```python
from build123d import *

# Parameters (mm, degrees)
F2_R     = 25.25
F3_DEPTH = 18
F4_R     = 23
F5_DEPTH = 2
F6_R     = 30.25
F6_R_2   = 25.25
F7_DEPTH = 12
F9_D     = 2
F9_DEPTH = 5
F9_TIP   = 0.600860619


with BuildPart() as f1:
    # F0 (on Right) → F1 (revolve)
    with BuildSketch(Plane.YZ):
        Polygon((0, 41), (0, 0), (20, 0), (20, 41), (16, 41), (16, 35), (12, 35), (6, 41), align=None)
    revolve(axis=Axis((0, 10, 0), (0, -1, 0)))

    # F2 (on face) → F3 (cut)
    with BuildSketch(Plane(origin=(0, 20, 0), x_dir=(-1, 0, 0), z_dir=(0, 1, 0))):
        Circle(F2_R)
    extrude(amount=-F3_DEPTH, mode=Mode.SUBTRACT)

    # F4 (on face) → F5 (cut, through all)
    with BuildSketch(Plane.XZ):
        Circle(F4_R)
    extrude(amount=-F5_DEPTH, mode=Mode.SUBTRACT)

    # F6 (on face) → F7 (cut)
    with BuildSketch(Plane(origin=(0, 20, 0), x_dir=(-1, 0, 0), z_dir=(0, 1, 0))):
        Circle(F6_R)
        Circle(F6_R_2, mode=Mode.SUBTRACT)
    extrude(amount=-F7_DEPTH, mode=Mode.SUBTRACT)

    # F9
    with Locations(Plane(origin=(0, 8, 0), x_dir=(-1, 0, 0), z_dir=(0, 1, 0))):
        with Locations((0, 27.75), (24.032204955, -13.875), (-24.032204955, -13.875)):
            Hole(F9_D / 2, depth=F9_DEPTH)
            with Locations((0, 0, -(F9_DEPTH + F9_TIP / 2))):  # 118° drill point
                Cone(0, F9_D / 2, F9_TIP, mode=Mode.SUBTRACT)


solid = f1.part
```
The listing builds one solid part. Answer for the finished solid, in the listing's coordinates (mm). A direction names the side the tool comes from. Give positions to 0.01 mm unless a question says otherwise; leave off trailing zeros. Order: outer loops, then holes, each group sorted by start corner. A loop starts at its lowest first (then second) coordinate and runs counter-clockwise, first axis right, second up. Notation, with made-up numbers: (22.25, 56.5) -> (72.25, 56.5) arc R14 ccw to (72.25, 62.5) -> close; hole circle Ø8 at (-12.5, -29). An arc over 180 degrees is marked (long way). One line per item, written item: value.
1) Flat-ended cylindrical pins translate along their axes: P1, Ø4, axis at x = 25.5, z = 3.5, coming from the +Y side; P2, Ø3, axis at x = 0, z = 27.75, coming from the -Y side; P3, Ø10, axis at y = 5.5, z = -8, coming from the +X side; P4, Ø10, axis at y = 11, z = 19, coming from the -X side. Find the tip coordinate at first contact, or state that the pin passes through.
Reported:
P1: stops at y = 8
P2: stops at y = 0
P3: stops at x = 40.89
P4: stops at x = -36.85
2) Find section A-A, the plane z = 0. Determine the outline of the cut face in (x, y), plus the area to 3 significant figures.
Reported:
outline: (-41, 0) -> (-23, 0) -> (-23, 2) -> (-25.25, 2) -> (-25.25, 8) -> (-30.25, 8) -> (-30.25, 20) -> (-41, 20) -> (-41, 16) -> (-35, 16) -> (-35, 12) -> (-41, 6) -> close; (23, 0) -> (41, 0) -> (41, 6) -> (35, 12) -> (35, 16) -> (41, 16) -> (41, 20) -> (30.25, 20) -> (30.25, 8) -> (25.25, 8) -> (25.25, 2) -> (23, 2) -> close
area: 435 mm^2
3) Find the intervals of material crossed by line 1 (Z direction, x = 0, y = 6.15); line 2 (Z direction, x = 0, y = 1.05); line 3 (X direction, y = 10.25, z = -22), in increasing order.
Reported:
line 1: z = -40.85 to -25.25, 25.25 to 26.75, 28.75 to 40.85
line 2: z = -41 to -23, 23 to 41
line 3: x = -29.44 to -20.76, 20.76 to 29.44
4) A tool of negligible diameter and unlimited length cuts with its end or side. For faces 4 (the flat face through (-18.4, 16, 30.2)), 5 (the cylindrical face through (23.815, 5.465, -14.851)), 6 (the cylindrical face through (40, 3, -9)), from which of +Z, -Z, +X, -X, +Y, -Y can it reach the whole face along a straight path? Write none if from no direction.
Reported:
face 4: none
face 5: +Y
face 6: +Y, -Y
5) Determine the mould class of faces 1 (the flat face through (27, 20, 15)), 2 (the cylindrical face through (-0.13, 5.46, 28.74)), 3 (the cylindrical face through (21, 14, -28)) for opening direction Z: pulls with the +Z half, pulls with the -Z half, needs draft (parallel to the pull), parting line crosses it, or undercut.
Reported:
face 1: needs draft
face 2: undercut
face 3: parting line crosses it
